Geometry: final body of the model. Coordinates: model frame, mm. Face numbers are marked on the shaded views. A direction names the side the tool comes from. Round coordinates to 2 decimals unless told otherwise and drop trailing zeros. Loops run counter-clockwise (first coordinate to the right, second up) from the corner with the lowest first, then second, coordinate; pieces in that order, holes last. Notation, with made-up numbers: M 46.5,-36.5 L 61.5,-36.5 A28 ccw 61.5,-15.5 Z; hole C -16,32.25 d7. An arc over 180 degrees is marked long. Write each question's results on one line, items separated by ' | '.
```python
from build123d import *

# Parameters (mm, degrees)
BOSS_EXTRUDE2_DEPTH = 5
SKETCH6_R           = 9
CUT_EXTRUDE1_DEPTH  = 58.130534293
FILLET2_R           = 1
SKETCH7_R           = 7.5
BOSS_EXTRUDE3_DEPTH = 40


with BuildPart() as part:
    # Sketch4 → Boss-Extrude2 (new body)
    with BuildSketch(Plane.XY):
        with BuildLine():
            Line((-54.898979486, -3), (-54.898979486, 3))
            Line((-54.898979486, 3), (-14.696938457, 3))
            ThreePointArc((-14.696938457, 3), (15, 0), (-14.696938457, -3))
            Line((-14.696938457, -3), (-54.898979486, -3))
        make_face()
    extrude(amount=BOSS_EXTRUDE2_DEPTH)

    # Sketch6 → Cut-Extrude1 (cut, through all)
    with BuildSketch(Plane.XY.offset(5)):
        Circle(SKETCH6_R)
    extrude(amount=-CUT_EXTRUDE1_DEPTH, mode=Mode.SUBTRACT)

    # Fillet2
    fillet2_edges = [part.edges().sort_by_distance(p)[0] for p in [
        (15, 0, 5),
        (15, 0, 0),
    ]]
    fillet(fillet2_edges, radius=FILLET2_R)

    # Sketch7 → Boss-Extrude3 (add)
    with BuildSketch(Plane.ZY.offset(54.898979486)):
        with Locations((2.528088008, 0)):
            Circle(SKETCH7_R)
    extrude(amount=-BOSS_EXTRUDE3_DEPTH)


solid = part.part
```
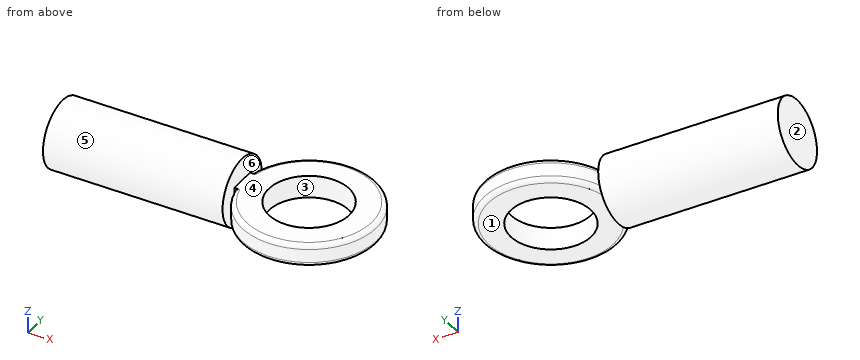
1. Draft query along X for the marked faces 1, 2 and 3. Return one class per face: pulls with the +X half, pulls with the -X half, needs draft (parallel to the pull), parting line crosses it, or undercut.
Answer key:
face 1: needs draft | face 2: pulls with the -X half | face 3: undercut
2. Pin query (flat end, axial travel): P1, Ø8.5, axis at x = -1, y = -6.5, coming from the -Z side; P2, Ø4, axis at x = 6.5, y = -9.5, coming from the +Z side; P3, Ø4, axis at x = -37, y = -8, coming from the -Z side. Return the tip coordinate at first contact, or that it passes through.
Answer key:
P1: stops at z = 0 | P2: stops at z = 5 | P3: stops at z = -1.97
3. Access query for the marked faces 4, 5 and 6. Directions: +Z, -Z, +X, -X, +Y, -Y. A direction counts if a zero-diameter tool reaches every point of the face in a straight line with its end or side. Return the directions, or none.
Answer key:
face 4: +Z, +X, +Y, -Y | face 5: -X | face 6: none
4. Ray query, probe 1 along Y at (x, z) = (0, 1.1); probe 2 along X at (y, z) = (2.5, -1); probe 3 along X at (y, z) = (12, 2.5). Return the intervals inside material, ascending.
Answer key:
probe 1: y = -15 to -9, 9 to 15 | probe 2: x = -54.9 to -14.9 | probe 3: x = -9 to 9
5. Section A-A (y = 0). Output: boundary loops of the cut face in (x, z), then the cut area to 3 significant figures.
Answer key:
outline: M -54.9,-4.97 L -14.9,-4.97 L -14.9,0 L -9,0 L -9,5 L -14.9,5 L -14.9,10.03 L -54.9,10.03 Z; M 9,0 L 14,0 A1 ccw 15,1 L 15,4 A1 ccw 14,5 L 9,5 Z | area: 659 mm²
6. Section B-B (z = 3.25). Output: boundary loops of the cut face in (x, y).
Answer key:
outline: M -54.9,-7.47 L -14.9,-7.47 L -14.9,-3 L -14.7,-3 A15 ccw long -14.7,3 L -14.9,3 L -14.9,7.47 L -54.9,7.47 Z; hole C 0,0 d18
7. Section C-C (x = -24.5). Output: boundary loops of the cut face in (y, z).
Answer key:
outline: C 0,2.53 d15
8. Section D-D (z = -3.25). Output: boundary loops of the cut face in (x, y).
Answer key:
outline: M -54.9,-4.78 L -14.9,-4.78 L -14.9,4.78 L -54.9,4.78 Z
